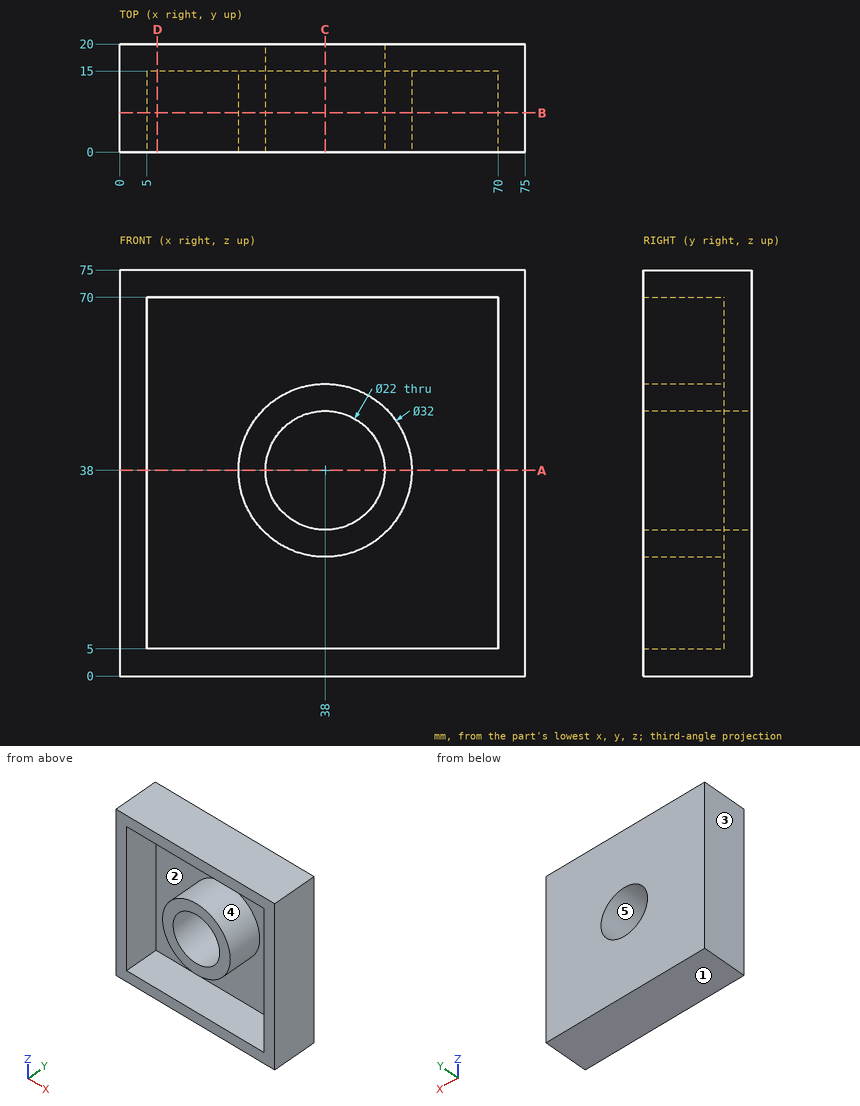
Check sheet for the drawn part. Datum: minimum x, y, z corner. Units: mm. A direction names the side the tool comes from. Round coordinates to 2 decimals unless told otherwise and drop trailing zeros. Write each loop counter-clockwise with the first axis right and the second up, starting at its lowest first coordinate (ties: lowest second). Pieces come first, ordered by that corner, then holes. Notation, with made-up numbers: (-11.75, -6.5) - (41.25, -6.5) arc R24 cw to (41.25, 12.5) - close; hole circle Ø2 at (18, -33). An arc over 180 degrees is marked (long way). Return JSON: item names as keys, results as strings.
Q1. Cross-section at A-A (z = 38). Record the boundary of the cut face in (x, y), then the cut area to 3 significant figures.
Returned:
{"outline": "(0, 0) - (5, 0) - (5, 15) - (22, 15) - (22, 0) - (27, 0) - (27, 20) - (0, 20) - close; (49, 0) - (54, 0) - (54, 15) - (70, 15) - (70, 0) - (75, 0) - (75, 20) - (49, 20) - close", "area": "565 mm²"}
Q2. Depth check by flat-ended pin: P1, Ø1, axis at x = 52.5, z = 11.5, coming from the -Y side; P2, Ø20, axis at x = 38, z = 38, coming from the -Y side. Enter the tip coordinate at first touch or a pass-through.
Returned:
{"P1": "stops at y = 15", "P2": "passes through"}
Q3. Scan lines: L1, parallel to X at y = 10.25, z = 38; L2, parallel to Z at x = 38, y = 15.25. Record each from-to range of solid material in increasing order. Write a range as from..to.
Returned:
{"L1": "x = 0..5, 22..27, 49..54, 70..75", "L2": "z = 0..27, 49..75"}
Q4. Cross-section at B-B (y = 7.25). Record the boundary of the cut face in (x, z).
Returned:
{"outline": "(0, 0) - (75, 0) - (75, 75) - (0, 75) - close; circle Ø32 at (38, 38); hole (5, 5) - (70, 5) - (70, 70) - (5, 70) - close; hole circle Ø22 at (38, 38)"}
Q5. Cross-section at C-C (x = 38). Record the boundary of the cut face in (y, z).
Returned:
{"outline": "(0, 0) - (20, 0) - (20, 27) - (0, 27) - (0, 22) - (15, 22) - (15, 5) - (0, 5) - close; (0, 49) - (20, 49) - (20, 75) - (0, 75) - (0, 70) - (15, 70) - (15, 54) - (0, 54) - close"}
Q6. Access from +Z, -Z, +X, -X, +Y, -Y to the whole of each face (thin tool, end or side, straight path). Record for the marked faces 4 and 5.
Returned:
{"face 4": "-Y", "face 5": "+Y, -Y"}
Q7. Cross-section at D-D (x = 7). Record the boundary of the cut face in (y, z).
Returned:
{"outline": "(0, 0) - (20, 0) - (20, 75) - (0, 75) - (0, 70) - (15, 70) - (15, 5) - (0, 5) - close"}
Q8. Draft check along X on the marked faces 1, 2 and 3. Enter one of: released by +X, released by -X, zero draft, split by the parting line, or undercut.
Returned:
{"face 1": "zero draft", "face 2": "undercut", "face 3": "released by -X"}
